Geometry check sheet. Reference: drawing and pictorial views, mm from the part's lowest x, y, z. Coordinates: 2 decimals unless noted, no trailing zeros. Order: outer loops, then holes, each group sorted by start corner. A loop starts at its lowest first (then second) coordinate and runs counter-clockwise, first axis right, second up. Notation, with made-up numbers: M 44,-30.5 L 79,-30.5 A7 ccw 79,-22.5 Z; hole C 21,20 d5. An arc over 180 degrees is marked long. Return JSON: item names as keys, results as strings.
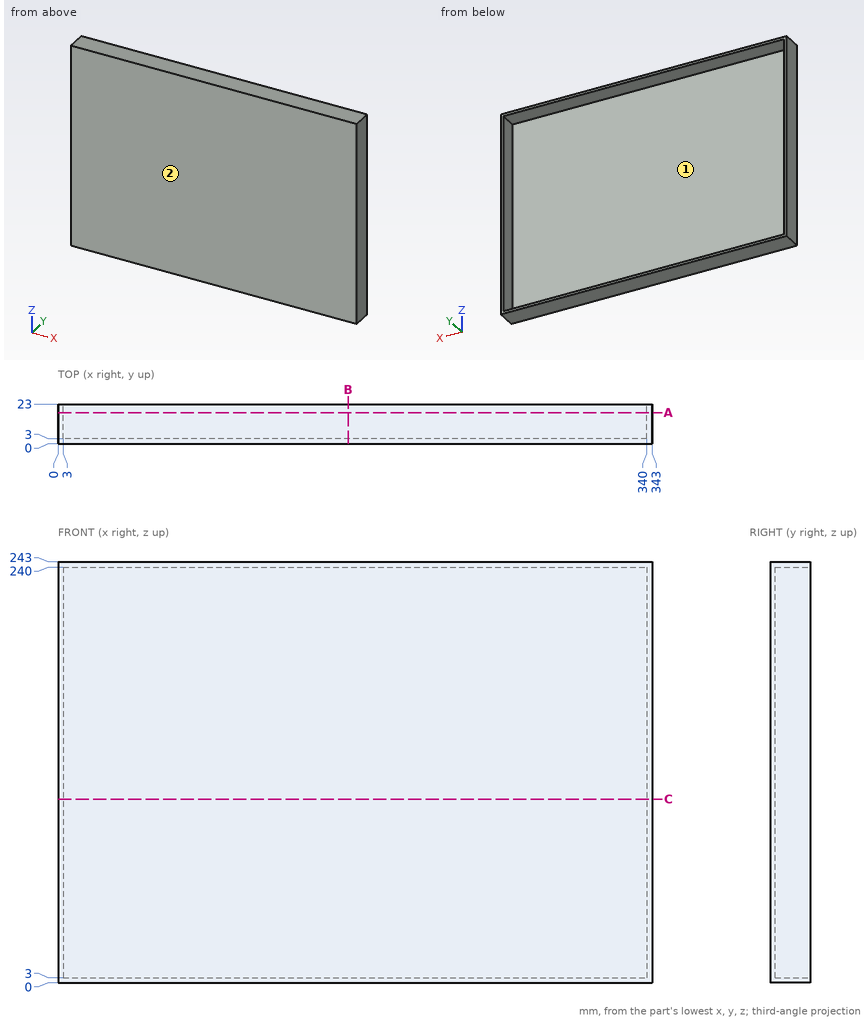
Q1. Cross-section at C-C, the plane z = 106. Record the boundary of the cut face in (x, y), and give its area (3 significant figures).
Values:
{"outline": "M 0,0 L 343,0 L 343,23 L 340,23 L 340,3 L 3,3 L 3,23 L 0,23 Z", "area": "1,150 mm^2"}
Q2. Go/stop test with a flat-tipped pin: pin 1 (3 mm diameter, centred on y = 9, z = 70.5, fed in from -X). Record where the tip stops, or that it passes through.
Values:
{"pin 1": "x = 0"}
Q3. Cross-section at A-A, the plane y = 18. Record the boundary of the cut face in (x, z), and give its area (3 significant figures).
Values:
{"outline": "M 0,0 L 343,0 L 343,243 L 0,243 Z; hole M 3,3 L 340,3 L 340,240 L 3,240 Z", "area": "3,480 mm^2"}
Q4. Cross-section at B-B, the plane x = 167.5. Record the boundary of the cut face in (y, z).
Values:
{"outline": "M 0,0 L 23,0 L 23,3 L 3,3 L 3,240 L 23,240 L 23,243 L 0,243 Z"}
Q5. Draft check along Z on the marked faces 1 and 2. Enter one of: pulls with the +Z half, pulls with the -Z half, needs draft (parallel to the pull), parting line crosses it, or undercut.
Values:
{"face 1": "undercut", "face 2": "needs draft"}
Q6. Material ranges on line 1 along X through (y, z) = (15.75, 190); line 2 along Z through (x, y) = (182, 7.5); line 3 along Y through (x, z) = (199, 218), recorded low to high.
Values:
{"line 1": "0 to 3, 340 to 343", "line 2": "0 to 3, 240 to 243", "line 3": "0 to 3"}
